Here's how the part is built. I have some questions about the finished solid (model axes, mm). Face numbers are marked on the shaded views. A direction names the side the tool comes from. Give positions to 0.01 mm unless a question says otherwise; leave off trailing zeros. Order: outer loops, then holes, each group sorted by start corner. A loop starts at its lowest first (then second) coordinate and runs counter-clockwise, first axis right, second up.
from build123d import *

# Parameters (mm, degrees)
SKETCH1_R               = 9.525
BASE_EXTRUDE_DEPTH      = 39.6875
CUT_EXTRUDE1_START      = -17.272
CUT_EXTRUDE1_DEPTH      = 17.272
CUT_EXTRUDE2_DEPTH      = 42.911202634
CUT_EXTRUDE2_DEPTH_BACK = 42.911202634
SKETCH3_R               = 3.175
CHAMFER1_SIZE           = 1.27


with BuildPart() as part:
    # Sketch1 → Base-Extrude (new body)
    with BuildSketch(Plane(origin=(0, 0, 0), x_dir=(0, 0, -1), z_dir=(1, 0, 0))):
        with Locations(Location((0, 0, 0), (0, 0, 180))):
            Circle(SKETCH1_R)
    extrude(amount=BASE_EXTRUDE_DEPTH)

    # Sketch2 → Cut-Extrude1 (cut)
    with BuildSketch(Plane(origin=(39.6875, 0, 0), x_dir=(0, 0, -1), z_dir=(1, 0, 0)).offset(CUT_EXTRUDE1_START)):
        with BuildLine():
            Line((-3.96875, 8.658790241), (-3.96875, -8.658790241))
            ThreePointArc((-3.96875, -8.658790241), (0, -9.525), (3.96875, -8.658790241))
            Line((3.96875, -8.658790241), (3.96875, 8.658790241))
            ThreePointArc((3.96875, 8.658790241), (0, 9.525), (-3.96875, 8.658790241))
        make_face()
    extrude(amount=CUT_EXTRUDE1_DEPTH, mode=Mode.SUBTRACT)

    # Sketch3 → Cut-Extrude2 (cut, two sides: drawn at the far end of the back side and taken through both)
    with BuildSketch(Plane.XY.offset(-CUT_EXTRUDE2_DEPTH_BACK)):
        with Locations((33.274, 0)):
            Circle(SKETCH3_R)
    extrude(amount=CUT_EXTRUDE2_DEPTH + CUT_EXTRUDE2_DEPTH_BACK, mode=Mode.SUBTRACT)

    # Chamfer1
    chamfer1_edges = [part.edges().sort_by_distance(p)[0] for p in [
        (0, 0, -9.525),
        (39.6875, -5.144087929, 8.016482045),
        (39.6875, 0, -9.525),
    ]]
    chamfer(chamfer1_edges, length=CHAMFER1_SIZE)


solid = part.part
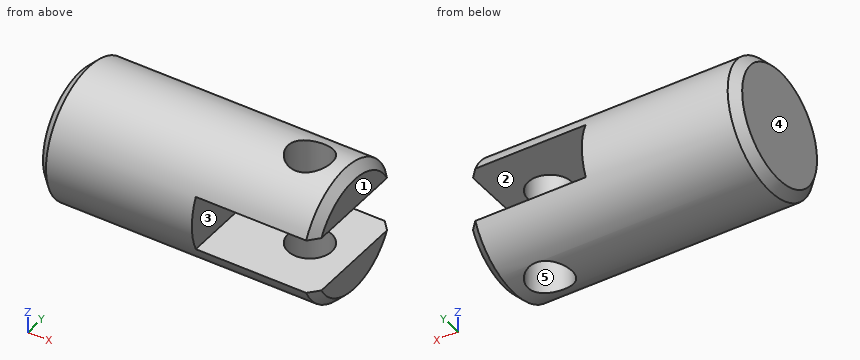
Q1. Thinking about a two-plate mould opening in X: for the marked faces 3, 4 and 5, which applies, released by +X, released by -X, zero draft, split by the parting line, or undercut?
Filled sheet:
face 3: released by +X
face 4: released by -X
face 5: undercut
Q2. If we section it at A-A on y = 0: List the corners of the cut face in (x, z) for me (1 decimal).
Filled sheet:
outline: (0, -8.3) - (1.3, -9.5) - (30.1, -9.5) - (30.1, -4) - (22.4, -4) - (22.4, 4) - (30.1, 4) - (30.1, 9.5) - (1.3, 9.5) - (0, 8.3) - close; (36.4, -9.5) - (38.4, -9.5) - (39.7, -8.3) - (39.7, -4) - (36.4, -4) - close; (36.4, 4) - (39.7, 4) - (39.7, 8.3) - (38.4, 9.5) - (36.4, 9.5) - close
Q3. If we section it at D-D on x = 13: List the corners of the cut face in (y, z) for me (3 decimals).
Filled sheet:
outline: circle Ø19.05 at (0, 0)
Q4. For the marked faces 1 and 2, which set-ups out of +Z, -Z, +X, -X, +Y, -Y let a thin tool reach every point of the face, with its end or its side?
Filled sheet:
face 1: +Z, -Z, +X, +Y, -Y
face 2: +X, +Y, -Y
Q5. If we section it at C-C on x = 32.5: List the corners of the cut face in (y, z) for me (3 decimals), plus the area to 3 significant figures.
Filled sheet:
outline: (-8.659, -3.969) arc R9.525 ccw to (-3.079, -9.014) - (-3.079, -3.969) - close; (-8.659, 3.969) - (-3.079, 3.969) - (-3.079, 9.014) arc R9.525 ccw to start; (3.079, -9.014) arc R9.525 ccw to (8.659, -3.969) - (3.079, -3.969) - close; (3.079, 3.969) - (8.659, 3.969) arc R9.525 ccw to (3.079, 9.014) - close
area: 72.0 mm2
Q6. If we section it at B-B on z = 0: List the corners of the cut face in (x, y) for me (1 decimal).
Filled sheet:
outline: (0, -8.3) - (1.3, -9.5) - (22.4, -9.5) - (22.4, 9.5) - (1.3, 9.5) - (0, 8.3) - close
Q7. I'm going to push flat-ended pins straight in: P1, Ø8, axis at x = 23.5, z = -3, coming from the +Y side (3 decimals); P2, Ø4, axis at x = 11, y = -6, coming from the -Z side; P3, Ø5.5, axis at x = 33.274, y = 0, coming from the +Z side; P4, Ø2, axis at x = 20.5, z = 7, coming from the -Y side. Where does each tip first touch, or does it pass through?
Filled sheet:
P1: stops at y = 9.525
P2: stops at z = -8.64
P3: passes through
P4: stops at y = -7.4
Q8. I need wall thicknesses on L1, parallel to X at y = 0, z = -5.1; L2, parallel to X at y = 1.75, z = 2.25; L3, parallel to Z at x = 35, y = 7.5. Which ranges of each line are inside material? Lowest first, please.
Filled sheet:
L1: x = 0 to 30.1, 36.45 to 39.69
L2: x = 0 to 22.42
L3: z = -5.87 to -3.97, 3.97 to 5.87
